For this review, take the finished solid that the model builds, in its own axes (mm). Round coordinates to 2 decimals unless told otherwise and drop trailing zeros. Write each loop counter-clockwise with the first axis right and the second up, starting at its lowest first coordinate (ties: lowest second). Pieces come first, ordered by that corner, then holes. Notation, with made-up numbers: (71.25, -31) - (104.25, -31) arc R15 cw to (104.25, -26) - close; hole circle Ø11 at (1, 77.5). An arc over 180 degrees is marked (long way). Answer in a Markdown table with one row per item. Add a question column.
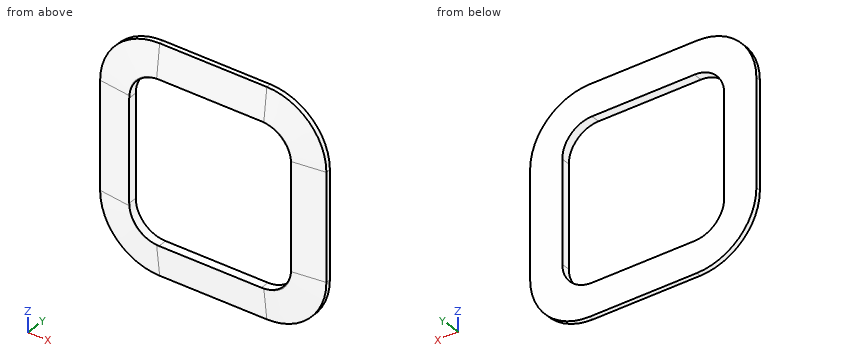
from build123d import *

# Parameters (mm, degrees)
SKETCH1_W      = 38
SKETCH1_H      = 38
SKETCH1_W_2    = 27.2
SKETCH1_H_2    = 27.2
EXTRUDE1_DEPTH = 1.5
FILLET1_R      = 5
FILLET2_R      = 10


with BuildPart() as part:
    # Sketch1 → Extrude1 (new body)
    with BuildSketch(Plane(origin=(0, 0, 0), x_dir=(1, 0, 0), z_dir=(0, 1, 0))):
        Rectangle(SKETCH1_W, SKETCH1_H)
        Rectangle(SKETCH1_W_2, SKETCH1_H_2, mode=Mode.SUBTRACT)
    extrude(amount=-EXTRUDE1_DEPTH)

    # Fillet1
    fillet1_edges = [part.edges().sort_by_distance(p)[0] for p in [
        (-13.6, -0.75, 13.6),
        (-13.6, -0.75, -13.6),
        (13.6, -0.75, -13.6),
        (13.6, -0.75, 13.6),
    ]]
    fillet(fillet1_edges, radius=FILLET1_R)

    # Fillet2
    fillet2_edges = [part.edges().sort_by_distance(p)[0] for p in [
        (-19, -0.75, -19),
        (19, -0.75, -19),
        (19, -0.75, 19),
        (-19, -0.75, 19),
    ]]
    fillet(fillet2_edges, radius=FILLET2_R)

    # Cut-Sweep1: sweep along a path in Sketch4
    with BuildLine(Plane.XZ.offset(1.5)) as cut_sweep1_path:
        Line((9, -19), (-9, -19))
        ThreePointArc((-9, -19), (-16.071067812, -16.071067812), (-19, -9))
        Line((-19, -9), (-19, 9))
        ThreePointArc((-19, 9), (-16.071067812, 16.071067812), (-9, 19))
        Line((-9, 19), (9, 19))
        ThreePointArc((9, 19), (16.071067812, 16.071067812), (19, 9))
        Line((19, 9), (19, -9))
        ThreePointArc((19, -9), (16.071067812, -16.071067812), (9, -19))
    # Sketch2 → Cut-Sweep1 (sweep, cut)
    with BuildSketch(Plane.XY):
        Polygon((19, -0.8), (19, -1.5), (13.6, -1.5), align=None)
    sweep(path=cut_sweep1_path.line, mode=Mode.SUBTRACT)


solid = part.part
Q1. Add section A-A on x = -4.5. State the section outline as (y, z) points, then the cut area to 3 significant figures.
Q2. To check wall thickness, follow probe 1 along X at (y, z) = (-0.45, 5.5); probe 2 along Z at (x, y) = (12, -0.65). State the ranges of each line that lie inside material, in increasing order.
Q3. Add section B-B on z = 4. State the section outline as (x, y) points, then the cut area to 3 significant figures.
Q4. Add section C-C on y = -0.25. State the section outline as (x, z) points.
Answer sheet:
| question | item | result |
|---|---|---|
| 1 | outline | (-1.5, -13.6) - (-0.8, -19) - (0, -19) - (0, -13.6) - close; (-1.5, 13.6) - (0, 13.6) - (0, 19) - (-0.8, 19) - close |
| 1 | area | 12.4 mm² |
| 2 | probe 1 | x = -19 to -13.6, 13.6 to 19 |
| 2 | probe 2 | z = -18.54 to -12.27, 12.27 to 18.54 |
| 3 | outline | (-19, -0.8) - (-13.6, -1.5) - (-13.6, 0) - (-19, 0) - close; (13.6, -1.5) - (19, -0.8) - (19, 0) - (13.6, 0) - close |
| 3 | area | 12.4 mm² |
| 4 | outline | (-19, -9) arc R10 ccw to (-9, -19) - (9, -19) arc R10 ccw to (19, -9) - (19, 9) arc R10 ccw to (9, 19) - (-9, 19) arc R10 ccw to (-19, 9) - close; hole (-13.6, -8.6) arc R5 ccw to (-8.6, -13.6) - (8.6, -13.6) arc R5 ccw to (13.6, -8.6) - (13.6, 8.6) arc R5 ccw to (8.6, 13.6) - (-8.6, 13.6) arc R5 ccw to (-13.6, 8.6) - close |
